Design review of the part built by this model. Coordinates are the model's own, in mm. Coordinates: 2 decimals unless noted, no trailing zeros. Write each loop counter-clockwise with the first axis right and the second up, starting at its lowest first coordinate (ties: lowest second). Pieces come first, ordered by that corner, then holes.
Q1. Clearance check with a flat-ended pin moving along its axis: pin 1 Ø3.5 at (x, y) = (788.83, 594.65) entering from +Z. State where the tip first meets the part, or that it passes through.
Q2. To check wall thickness, follow probe 1 along X at (y, z) = (590, 0.85); probe 2 along Y at (x, z) = (777.5, 1.15); probe 3 along Y at (x, z) = (781, 0.5). State the ranges of each line that lie inside material, in increasing order.
Q3. Add section B-B, the plane x = 788. Give the boundary of the cut face in (y, z).
Q4. Add section C-C, the plane y = 594. Give the boundary of the cut face in (x, z).
Q5. Add section D-D, the plane y = 581.5. Give the boundary of the cut face in (x, z).
Q6. Add section A-A, the plane y = 572. Give the boundary of the cut face in (x, z).
from build123d import *

# Parameters (mm, degrees)
MODEL_R         = 2
MODEL_W         = 10
MODEL_H         = 2
MODEL_W_2       = 4.987831099
MODEL_H_2       = 25.799348384
EXTRUDE_1_DEPTH = 2


with BuildPart() as part:
    # Model → 凸台-拉伸1 (new body)
    with BuildSketch(Plane.XY):
        Polygon((794.826364885, 604.086609439), (759.826364885, 604.086609439), (759.826364885, 582.631162925), (771.100956458, 576.121774445), (771.100956458, 571.121774445), (765.159330178, 567.691374913), (765.159330178, 566.808009524), (762.184594735, 566.808009524), (765.159330178, 564.224720814), (762.184594735, 564.224720814), (765.159330178, 561.641432105), (762.184594735, 561.641432105), (765.159330178, 559.256659904), (789.493399591, 559.256659904), (792.468135034, 561.641432105), (789.493399591, 561.641432105), (792.468135034, 564.224720814), (789.493399591, 564.224720814), (792.468135034, 566.808009524), (789.493399591, 566.808009524), (789.493399591, 567.691374913), (783.551773312, 571.121774445), (783.551773312, 576.121774445), (794.826364885, 582.631162925), align=None)
        with Locations((765.826364885, 594.647306527)):
            Circle(MODEL_R, mode=Mode.SUBTRACT)
        with Locations((788.826364885, 594.647306527)):
            Circle(MODEL_R, mode=Mode.SUBTRACT)
        with Locations((784.826364885, 589.647718545)):
            Rectangle(MODEL_W, MODEL_H, mode=Mode.SUBTRACT)
        with Locations((769.826364885, 589.647718545)):
            Rectangle(MODEL_W, MODEL_H, mode=Mode.SUBTRACT)
        Polygon((791.725011171, 587.146217285), (781.894706262, 587.146217285), (781.894706262, 578.118128773), (791.725011171, 583.659501515), align=None, mode=Mode.SUBTRACT)
        with Locations((777.326364885, 574.246543093)):
            Rectangle(MODEL_W_2, MODEL_H_2, mode=Mode.SUBTRACT)
        Polygon((787.11688102, 566.27157462), (782.629496351, 568.945406022), (781.869533608, 568.945406022), (781.869533608, 561.448894487), (787.11688102, 561.448894487), align=None, mode=Mode.SUBTRACT)
        Polygon((762.927718599, 587.146217285), (772.758023508, 587.146217285), (772.758023508, 578.118128773), (762.927718599, 583.659501515), align=None, mode=Mode.SUBTRACT)
        Polygon((767.53584875, 566.27157462), (772.023233419, 568.945406022), (772.783196161, 568.945406022), (772.783196161, 561.448894487), (767.53584875, 561.448894487), align=None, mode=Mode.SUBTRACT)
        Polygon((782.896259254, 598.074237023), (782.886259254, 598.208237023), (782.866259254, 598.343237023), (782.836259254, 598.476237023), (782.786259254, 598.608237023), (782.726259254, 598.740237023), (782.646259254, 598.869237023), (782.566259254, 598.997237023), (782.466259254, 599.122237023), (782.346259254, 599.245237023), (782.226259254, 599.365237023), (782.086259254, 599.483237023), (781.936259254, 599.596237023), (781.776259254, 599.706237023), (781.606259254, 599.812237023), (781.426259254, 599.914237023), (781.236259254, 600.011237023), (781.036259254, 600.104237023), (780.826259254, 600.192237023), (780.606259254, 600.275237023), (780.376259254, 600.352237023), (780.146259254, 600.424237023), (779.896259254, 600.490237023), (779.656259254, 600.551237023), (779.396259254, 600.605237023), (779.136259254, 600.654237023), (778.876259254, 600.696237023), (778.606259254, 600.732237023), (778.336259254, 600.761237023), (778.066259254, 600.784237023), (777.786259254, 600.801237023), (777.506259254, 600.810237023), (777.236259254, 600.814237023), (776.956259254, 600.810237023), (776.676259254, 600.801237023), (776.396259254, 600.784237023), (776.126259254, 600.761237023), (775.856259254, 600.732237023), (775.586259254, 600.696237023), (775.326259254, 600.654237023), (775.066259254, 600.605237023), (774.806259254, 600.551237023), (774.566259254, 600.490237023), (774.316259254, 600.424237023), (774.086259254, 600.352237023), (773.856259254, 600.275237023), (773.636259254, 600.192237023), (773.426259254, 600.104237023), (773.226259254, 600.011237023), (773.036259254, 599.914237023), (772.856259254, 599.812237023), (772.686259254, 599.706237023), (772.526259254, 599.596237023), (772.376259254, 599.483237023), (772.236259254, 599.365237023), (772.116259254, 599.245237023), (771.996259254, 599.122237023), (771.896259254, 598.997237023), (771.816259254, 598.869237023), (771.736259254, 598.740237023), (771.676259254, 598.608237023), (771.626259254, 598.476237023), (771.596259254, 598.343237023), (771.576259254, 598.208237023), (771.566259254, 598.074237023), (771.576259254, 597.940237023), (771.596259254, 597.805237023), (771.626259254, 597.672237023), (771.676259254, 597.540237023), (771.736259254, 597.408237023), (771.816259254, 597.279237023), (771.896259254, 597.151237023), (771.996259254, 597.026237023), (772.116259254, 596.903237023), (772.236259254, 596.783237023), (772.376259254, 596.666237023), (772.526259254, 596.552237023), (772.686259254, 596.442237023), (772.856259254, 596.336237023), (773.036259254, 596.234237023), (773.226259254, 596.137237023), (773.426259254, 596.044237023), (773.636259254, 595.956237023), (773.856259254, 595.873237023), (774.086259254, 595.796237023), (774.316259254, 595.724237023), (774.566259254, 595.658237023), (774.806259254, 595.597237023), (775.066259254, 595.543237023), (775.326259254, 595.494237023), (775.586259254, 595.452237023), (775.856259254, 595.416237023), (776.126259254, 595.387237023), (776.396259254, 595.364237023), (776.676259254, 595.347237023), (776.956259254, 595.338237023), (777.236259254, 595.334237023), (777.506259254, 595.338237023), (777.786259254, 595.347237023), (778.066259254, 595.364237023), (778.336259254, 595.387237023), (778.606259254, 595.416237023), (778.876259254, 595.452237023), (779.136259254, 595.494237023), (779.396259254, 595.543237023), (779.656259254, 595.597237023), (779.896259254, 595.658237023), (780.146259254, 595.724237023), (780.376259254, 595.796237023), (780.606259254, 595.873237023), (780.826259254, 595.956237023), (781.036259254, 596.044237023), (781.236259254, 596.137237023), (781.426259254, 596.234237023), (781.606259254, 596.336237023), (781.776259254, 596.442237023), (781.936259254, 596.552237023), (782.086259254, 596.666237023), (782.226259254, 596.783237023), (782.346259254, 596.903237023), (782.466259254, 597.026237023), (782.566259254, 597.151237023), (782.646259254, 597.279237023), (782.726259254, 597.408237023), (782.786259254, 597.540237023), (782.836259254, 597.672237023), (782.866259254, 597.805237023), (782.886259254, 597.940237023), align=None, mode=Mode.SUBTRACT)
    extrude(amount=EXTRUDE_1_DEPTH)


solid = part.part
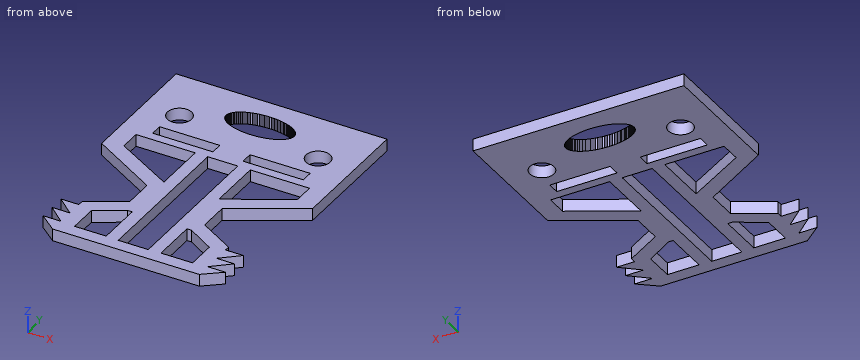
Here are the results:
1. pin 1: passes through
2. probe 1: x = 759.83 to 764.83, 774.83 to 779.83, 789.83 to 794.83
2. probe 2: y = 559.26 to 561.35, 587.15 to 595.34, 600.81 to 604.09
2. probe 3: y = 559.26 to 588.65, 590.65 to 596.03, 600.12 to 604.09
3. outline: (559.26, 0) - (568.55, 0) - (568.55, 2) - (559.26, 2) - close; (578.69, 0) - (581.56, 0) - (581.56, 2) - (578.69, 2) - close; (587.15, 0) - (588.65, 0) - (588.65, 2) - (587.15, 2) - close; (590.65, 0) - (592.83, 0) - (592.83, 2) - (590.65, 2) - close; (596.47, 0) - (604.09, 0) - (604.09, 2) - (596.47, 2) - close
4. outline: (759.83, 0) - (763.93, 0) - (763.93, 2) - (759.83, 2) - close; (767.72, 0) - (786.93, 0) - (786.93, 2) - (767.72, 2) - close; (790.72, 0) - (794.83, 0) - (794.83, 2) - (790.72, 2) - close
5. outline: (761.79, 0) - (766.76, 0) - (766.76, 2) - (761.79, 2) - close; (772.76, 0) - (774.83, 0) - (774.83, 2) - (772.76, 2) - close; (779.82, 0) - (781.89, 0) - (781.89, 2) - (779.82, 2) - close; (787.89, 0) - (792.87, 0) - (792.87, 2) - (787.89, 2) - close
6. outline: (771.1, 0) - (774.83, 0) - (774.83, 2) - (771.1, 2) - close; (779.82, 0) - (783.55, 0) - (783.55, 2) - (779.82, 2) - close
